Can you work these out from the model? Positions are in its coordinate system, mm. A direction names the side the tool comes from. Coordinates: 2 decimals unless noted, no trailing zeros. Answer as CSV lines item,"result". Start each with the question number.
1. If we section it at A-A (z = 5.25): Give the number of separate pieces and of enclosed holes in the cut face, plus the area to 3 significant figures.
2. If we mould it in two halves opening along X, with no side actions, what happens to faces 1 (the face through (163.112, 267.215, 5.437)), 2 (the face through (146, 259.88, 5)), 3 (the face through (173.56, 263.15, 4.93)), 4 (the face through (146, 251, 11))? For each: released by +X, released by -X, zero draft, split by the parting line, or undercut.
3. Will these pins go through, and if not, where does the flat tip stop? pin 1 (5 mm diameter, centred on y = 187.5, z = 9.5, fed in from +X); pin 2 (1.5 mm diameter, centred on x = 152, z = 3, fed in from -Y); pin 3 (6 mm diameter, centred on y = 185, z = 4.5, fed in from -X).
4. I need wall thicknesses on line 1 along Y through (x, z) = (147.5, 6.5) (3 decimals); line 2 along Y through (x, z) = (144, 0.75); line 3 along X through (y, z) = (237.5, 5.75). Which ranges of each line are inside material? Lowest first, please. Write a range as from..to.
5. On a 3-axis mill with a long thin cutter (end or side, diameter ignored), from which of +Z, -Z, +X, -X, +Y, -Y can I reach the whole of each face in a straight line? I mean faces 5 (the face through (147.147, 165.479, 10.584)), 6 (the face through (128.733, 267.211, 0.826)), 7 (the face through (128.906, 267.545, 5.437)). Say none if no direction works.
```python
from build123d import *

# Parameters (mm, degrees)
SKETCH001_R     = 37.5
SKETCH001_R_2   = 8
SKETCH001_R_3   = 1.25
PAD_DEPTH       = 11
CHAMFER_SIZE    = 1
CHAMFER001_SIZE = 1
FILLET_R        = 1
CHAMFER002_SIZE = 0.2
CHAMFER003_SIZE = 1


with BuildPart() as part:
    # Sketch001 → Pad (new body)
    with BuildSketch(Plane.XY):
        with BuildLine():
            ThreePointArc((160.234719, 302.98721), (146.009323, 313.229259), (131.783927, 302.98721))
            Line((104.755674, 222.17773), (131.783927, 302.98721))
            ThreePointArc((104.755674, 222.17773), (146.009323, 164.87967), (187.262972, 222.17773))
            Line((160.234719, 302.98721), (187.262972, 222.17773))
        make_face()
        with Locations((146.009323, 208.37967)):
            Circle(SKETCH001_R, mode=Mode.SUBTRACT)
        with Locations((146.009323, 298.229259)):
            Circle(SKETCH001_R_2, mode=Mode.SUBTRACT)
        with Locations((155.968615, 303.979259)):
            Circle(SKETCH001_R_3, mode=Mode.SUBTRACT)
        with Locations((146.009323, 286.729259)):
            Circle(SKETCH001_R_3, mode=Mode.SUBTRACT)
        with Locations((136.050031, 303.979259)):
            Circle(SKETCH001_R_3, mode=Mode.SUBTRACT)
        with Locations((146.009323, 248.87967)):
            Circle(SKETCH001_R_3, mode=Mode.SUBTRACT)
        with Locations((186.509323, 208.37967)):
            Circle(SKETCH001_R_3, mode=Mode.SUBTRACT)
        with Locations((146.009323, 167.87967)):
            Circle(SKETCH001_R_3, mode=Mode.SUBTRACT)
        with Locations((105.509323, 208.37967)):
            Circle(SKETCH001_R_3, mode=Mode.SUBTRACT)
        with BuildLine():
            ThreePointArc((136.404664, 274.87967), (128.904664, 267.37967), (136.404664, 259.87967))
            Line((136.404664, 259.87967), (155.613982, 259.87967))
            ThreePointArc((155.613982, 259.87967), (163.113982, 267.37967), (155.613982, 274.87967))
            Line((136.404664, 274.87967), (155.613982, 274.87967))
        make_face(mode=Mode.SUBTRACT)
    extrude(amount=PAD_DEPTH)

    # Chamfer
    chamfer_edges = [part.edges().sort_by_distance(p)[0] for p in [
        (108.509323, 208.37967, 11),
        (146.009323, 274.87967, 0),
    ]]
    chamfer(chamfer_edges, length=CHAMFER_SIZE)

    # Chamfer001
    chamfer001_edges = [part.edges().sort_by_distance(p)[0] for p in [
        (173.748846, 262.58247, 11),
    ]]
    chamfer(chamfer001_edges, length=CHAMFER001_SIZE)

    # Fillet
    fillet_edges = [part.edges().sort_by_distance(p)[0] for p in [
        (146.009323, 274.87967, 11),
        (107.509323, 208.37967, 11),
        (119.21816, 262.265273, 11),
        (146.009323, 165.87967, 11),
    ]]
    fillet(fillet_edges, radius=FILLET_R)

    # Chamfer002
    chamfer002_edges = [part.edges().sort_by_distance(p)[0] for p in [
        (144.759323, 286.729259, 11),
        (134.800031, 303.979259, 11),
        (154.718615, 303.979259, 11),
        (185.259323, 208.37967, 11),
        (144.759323, 167.87967, 11),
        (104.259323, 208.37967, 11),
        (144.759323, 248.87967, 11),
    ]]
    chamfer(chamfer002_edges, length=CHAMFER002_SIZE)

    # Chamfer003
    chamfer003_edges = [part.edges().sort_by_distance(p)[0] for p in [
        (138.009323, 298.229259, 11),
    ]]
    chamfer(chamfer003_edges, length=CHAMFER003_SIZE)


solid = part.part
```
Solved:
1,separate pieces,"1"
1,enclosed holes,"10"
1,area,"3,730 mm²"
2,face 1,"undercut"
2,face 2,"undercut"
2,face 3,"released by +X"
2,face 4,"zero draft"
3,pin 1,"x = 185.44"
3,pin 2,"y = 165.2"
3,pin 3,"x = 107.58"
4,line 1,"164.905..170.909, 245.85..259.88, 274.88..290.369, 306.089..313.155"
4,line 2,"164.93..170.93, 245.83..259.63, 275.13..290.49, 305.97..313.09"
4,line 3,"109.88..122.38, 169.64..182.14"
5,face 5,"+Z"
5,face 6,"-Z"
5,face 7,"+Z, -Z"
